Here's the drawing with two shaded views (mm, measured from the low corner). I have some questions. Give positions to 0.01 mm unless a question says otherwise; leave off trailing zeros. Loops run counter-clockwise (first coordinate to the right, second up) from the corner with the lowest first, then second, coordinate; pieces in that order, holes last. Notation, with made-up numbers: (20.5, -14.5) -> (41.5, -14.5) arc R23 ccw to (41.5, 14.5) -> close; hole circle Ø5 at (15, -6.75). An arc over 180 degrees is marked (long way). Put each result on its own line as item: value.
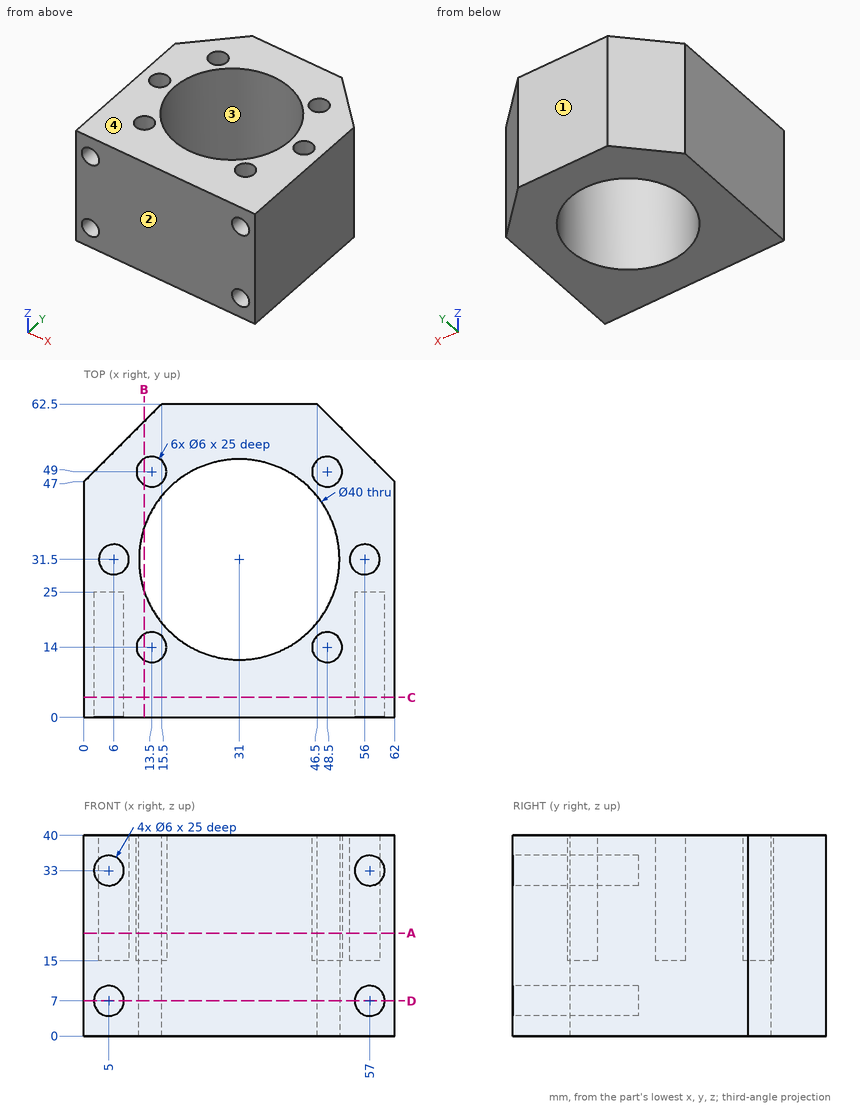
1. Thinking about a two-plate mould opening in Y: for the marked faces 1, 2, 3 and 4, which applies, pulls with the +Y half, pulls with the -Y half, needs draft (parallel to the pull), parting line crosses it, or undercut?
Recorded:
face 1: pulls with the +Y half
face 2: pulls with the -Y half
face 3: undercut
face 4: needs draft
2. If we section it at B-B (x = 12): List the corners of the cut face in (y, z) for me (3 decimals), then the cut area to 3 significant figures.
Recorded:
outline: (0, 0) -> (25.255, 0) -> (25.255, 40) -> (16.598, 40) -> (16.598, 15) -> (11.402, 15) -> (11.402, 40) -> (0, 40) -> close; (37.745, 0) -> (59, 0) -> (59, 40) -> (51.598, 40) -> (51.598, 15) -> (46.402, 15) -> (46.402, 40) -> (37.745, 40) -> close
area: 1,600 mm^2
3. If we section it at C-C (y = 4): List the corners of the cut face in (x, z) for me, then the cut area to 3 significant figures.
Recorded:
outline: (0, 0) -> (62, 0) -> (62, 40) -> (0, 40) -> close; hole circle Ø6 at (5, 7); hole circle Ø6 at (5, 33); hole circle Ø6 at (57, 7); hole circle Ø6 at (57, 33)
area: 2,370 mm^2
4. If we section it at A-A (z = 20.5): List the corners of the cut face in (x, y) for me, then the cut area to 3 significant figures.
Recorded:
outline: (0, 0) -> (62, 0) -> (62, 47) -> (46.5, 62.5) -> (15.5, 62.5) -> (0, 47) -> close; hole circle Ø6 at (6, 31.5); hole circle Ø6 at (13.5, 14); hole circle Ø6 at (13.5, 49); hole circle Ø40 at (31, 31.5); hole circle Ø6 at (48.5, 14); hole circle Ø6 at (48.5, 49); hole circle Ø6 at (56, 31.5)
area: 2,210 mm^2
5. If we section it at D-D (z = 7): List the corners of the cut face in (x, y) for me.
Recorded:
outline: (0, 0) -> (2, 0) -> (2, 25) -> (8, 25) -> (8, 0) -> (54, 0) -> (54, 25) -> (60, 25) -> (60, 0) -> (62, 0) -> (62, 47) -> (46.5, 62.5) -> (15.5, 62.5) -> (0, 47) -> close; hole circle Ø40 at (31, 31.5)
6. I need wall thicknesses on line 1 (Z direction, x = 5, y = 10); line 2 (Y direction, x = 48.5, z = 24); line 3 (Y direction, x = 47, z = 35). Which ranges of each line are inside material? Lowest first, please.
Recorded:
line 1: z = 0 to 4, 10 to 30, 36 to 40
line 2: y = 0 to 11, 17 to 21.82, 41.18 to 46, 52 to 60.5
line 3: y = 0 to 11.4, 16.6 to 19.5, 43.5 to 46.4, 51.6 to 62
7. I'm going to push flat-ended pins straight in: pin 1 (1 mm diameter, centred on x = 45.5, z = 9.5, fed in from -Y); pin 2 (1.8 mm diameter, centred on x = 56.5, z = 6, fed in from -Y); pin 3 (1.8 mm diameter, centred on x = 12.5, y = 48, fed in from +Z); pin 4 (7 mm diameter, centred on x = 5, z = 33, fed in from +Y). Where does each tip first touch, or does it pass through?
Recorded:
pin 1: stops at y = 0
pin 2: stops at y = 25
pin 3: stops at z = 15
pin 4: stops at y = 55.5
